from build123d import *

# Parameters (mm, degrees)
SKETCH1_W                      = 50.8
SKETCH1_H                      = 25.4
BOSS_EXTRUDE1_DEPTH            = 25.4
SKETCH2_W                      = 22.225
SKETCH2_H                      = 22.225
CUT_EXTRUDE1_DEPTH             = 86.194189943
F_7_0_201_DIAMETER_HOLE1_D     = 5.1054
F_7_0_201_DIAMETER_HOLE1_DEPTH = 25.4
F_7_0_201_DIAMETER_HOLE2_D     = 5.1054


with BuildPart() as part:
    # Sketch1 → Boss-Extrude1 (new body)
    with BuildSketch(Plane(origin=(0, 63.5, 0), x_dir=(1, 0, 0), z_dir=(0, 1, 0))):
        with Locations((25.4, -12.7)):
            Rectangle(SKETCH1_W, SKETCH1_H)
    extrude(amount=-BOSS_EXTRUDE1_DEPTH)

    # Sketch2 → Cut-Extrude1 (cut, through all)
    with BuildSketch(Plane(origin=(50.8, 0, 0), x_dir=(0, 0, -1), z_dir=(1, 0, 0))):
        with Locations((-14.2875, 52.3875)):
            Rectangle(SKETCH2_W, SKETCH2_H)
    extrude(amount=-CUT_EXTRUDE1_DEPTH, mode=Mode.SUBTRACT)

    # #7 (0.201) Diameter Hole1
    with Locations(Plane.XZ.offset(-38.1)):
        with Locations((-12.7, -12.7), (38.1, 12.7)):
            Hole(F_7_0_201_DIAMETER_HOLE1_D / 2, depth=F_7_0_201_DIAMETER_HOLE1_DEPTH)

    # #7 (0.201) Diameter Hole2 (through all)
    with Locations(Plane.XY.offset(3.175)):
        with Locations((38.1, 50.8), (12.7, 50.8)):
            Hole(F_7_0_201_DIAMETER_HOLE2_D / 2)


solid = part.part
For this review, take the finished solid that the model builds, in its own axes (mm). Give positions to 0.01 mm unless a question says otherwise; leave off trailing zeros. Order: outer loops, then holes, each group sorted by start corner. A loop starts at its lowest first (then second) coordinate and runs counter-clockwise, first axis right, second up. Notation, with made-up numbers: M 41,-37 L 79,-37 A7 ccw 79,-30 Z; hole C -39.5,37.25 d2. An arc over 180 degrees is marked long. Answer in a Markdown table with one row per item. Add a question column.
(1) For pin 1 (1 mm diameter, centred on x = 11.5, z = 17.5, fed in from +Y) (3 decimals); pin 2 (8 mm diameter, centred on x = 27, y = 51, fed in from +Z) (3 decimals), all flat-tipped, find the tip position at first contact; note any pin that passes through.
(2) Consider section D-D on x = 13.5. State the section outline as (y, z) points (3 decimals), and give its area (3 significant figures).
(3) Wall thickness on probe 1 along Z at (x, y) = (38.1, 40); probe 2 along Y at (x, z) = (38.1, 1.4); probe 3 along X at (y, z) = (52.5, 2.5): over which ranges is each line inside the solid? List them lowest first. Write a range as [from, to].
(4) Consider section C-C on z = 12.7. State the section outline as (x, y) points (3 decimals), and give its area (3 significant figures).
(5) Consider section B-B on x = 38.1. State the section outline as (y, z) points (3 decimals), and give its area (3 significant figures).
(6) Mouldability with a two-part tool opening along Y and no side actions: class faces 1 (the face through (38.43, 53.33, 1.57)), 2 (the face through (13.03, 53.33, 1.57)), 3 (the face through (26, 52, 3.175)), 4 (the face through (26, 41.275, 14)) as +Y half, -Y half, draft (parallel to the pull), parting line (faces both ways), or undercut.
(7) Consider section A-A on y = 50.8. State the section outline as (x, z) points (3 decimals).
Evaluation:
| question | item | result |
|---|---|---|
| 1 | pin 1 | stops at y = 41.275 |
| 1 | pin 2 | stops at z = 3.175 |
| 2 | outline | M 38.1,0 L 48.376,0 L 48.376,3.175 L 41.275,3.175 L 41.275,25.4 L 38.1,25.4 Z; M 53.224,0 L 63.5,0 L 63.5,3.175 L 53.224,3.175 Z |
| 2 | area | 136 mm^2 |
| 3 | probe 1 | z = [0, 10.15], [15.25, 25.4] |
| 3 | probe 2 | y = [38.1, 48.25], [53.35, 63.5] |
| 3 | probe 3 | x = [0, 10.8], [14.6, 36.2], [40, 50.8] |
| 4 | outline | M 0,38.1 L 35.547,38.1 L 35.547,41.275 L 0,41.275 Z; M 40.653,38.1 L 50.8,38.1 L 50.8,41.275 L 40.653,41.275 Z |
| 4 | area | 145 mm^2 |
| 5 | outline | M 38.1,0 L 48.247,0 L 48.247,3.175 L 41.275,3.175 L 41.275,10.147 L 38.1,10.147 Z; M 38.1,15.253 L 41.275,15.253 L 41.275,25.4 L 38.1,25.4 Z; M 53.353,0 L 63.5,0 L 63.5,3.175 L 53.353,3.175 Z |
| 5 | area | 119 mm^2 |
| 6 | face 1 | undercut |
| 6 | face 2 | undercut |
| 6 | face 3 | draft |
| 6 | face 4 | +Y half |
| 7 | outline | M 0,0 L 10.147,0 L 10.147,3.175 L 0,3.175 Z; M 15.253,0 L 35.547,0 L 35.547,3.175 L 15.253,3.175 Z; M 40.653,0 L 50.8,0 L 50.8,3.175 L 40.653,3.175 Z |
